Geometry: final body of the model. Coordinates: model frame, mm. A direction names the side the tool comes from. Give positions to 0.01 mm unless a question says otherwise; leave off trailing zeros. Write each loop counter-clockwise with the first axis right and the second up, starting at its lowest first coordinate (ties: lowest second). Pieces come first, ordered by that corner, then holes. Notation, with made-up numbers: (6.5, -7) -> (29.5, -7) arc R24 ccw to (29.5, 27) -> close; hole circle Ø2 at (11.5, -37.75). An arc over 180 degrees is marked (long way). Answer in a Markdown table with one row per item. Add a question column.
Item 1: Draft query along Y for faces 4 (the flat face through (-7.482, 2.799, 0.246)), 5 (the cylindrical face through (-7.956, 7.296, 0.682)), 6 (the flat face through (0, 0, 5)). Return one class per face: +Y half, -Y half, draft (parallel to the pull), parting line (faces both ways), or undercut.
Item 2: Material intervals for probe 1 along Z at (x, y) = (-5.25, 7.25); probe 2 along Z at (x, y) = (6, 2); probe 3 along X at (y, z) = (2.25, 3.9), sorted ascending. Write a range as from..to.
Item 3: Section query B-B on z = 3.6. Output: boundary loops of the cut face in (x, y).
Item 4: Section query A-A on y = 0. Output: boundary loops of the cut face in (x, z) (3 decimals), plus the area to 3 significant figures.
Item 5: First-contact query: P1, Ø1.5, axis at x = -5.5, y = -5, coming from the +Z side; P2, Ø11.5, axis at x = 4.5, y = -1, coming from the -Z side; P3, Ø1.5, axis at y = 2, z = 2, coming from the -X side; P4, Ø3, axis at x = -6.5, z = 0.5, coming from the +Y side. Flat tips, straight axial feed; report the tip coordinate or a pass-through.
Item 6: Access query for faces 1 (the flat face through (0, 0, 0)), 2 (the flat face through (-1.387, -4.757, 0.246)), 3 (the flat face through (2, -4, 2.5)). Directions: +Z, -Z, +X, -X, +Y, -Y. A direction counts if a zero-diameter tool reaches every point of the face in a straight line with its end or side. Return the directions, or none.
```python
from build123d import *

# Parameters (mm, degrees)
F0_R     = 4.064
F1_DEPTH = 5
F0_R_2   = 8.89
F2_DEPTH = 2.5
F0_R_3   = 10.795
F3_DEPTH = 1.5
F5_DEPTH = 0.5
F6_SIZE  = 0.508
F7_SIZE  = 0.381


with BuildPart() as f1:
    # F0 (on Top) → F1 (new body)
    with BuildSketch(Plane.XY):
        Circle(F0_R)
    extrude(amount=F1_DEPTH)

    # F0 (on Top) → F2 (join)
    with BuildSketch(Plane.XY):
        Circle(F0_R_2)
        Circle(F0_R, mode=Mode.SUBTRACT)
    extrude(amount=F2_DEPTH)

    # F0 (on Top) → F3 (join)
    with BuildSketch(Plane.XY):
        Circle(F0_R_3)
        Circle(F0_R_2, mode=Mode.SUBTRACT)
    extrude(amount=F3_DEPTH)

    # F4 (on face) → F5 (cut)
    with BuildSketch(Plane(origin=(0, 0, 0), x_dir=(1, 0, 0), z_dir=(0, 0, -1))):
        Polygon((-6.200742, -0.58), (-8.798818, -5.08), (-1.75, -5.08), (-1.75, -3.58), (-6.200742, -3.58), (-4.468691, -0.58), align=None)
        Polygon((0, 10.16), (-5.334716, 0.92), (-3.602666, 0.92), (-2.73664, 2.42), (0, 7.16), (1.870615, 3.92), (3.602666, 3.92), align=None)
        Polygon((1.75, -3.58), (1.75, -5.08), (8.798818, -5.08), (4.468691, 2.42), (2.73664, 2.42), (3.602666, 0.92), (6.200742, -3.58), align=None)
        Polygon((-2.73664, 2.42), (-3.602666, 0.92), (3.602666, 0.92), (2.73664, 2.42), align=None)
    extrude(amount=-F5_DEPTH, mode=Mode.SUBTRACT)

    # F6
    f6_edges = [f1.edges().sort_by_distance(p)[0] for p in [
        (-10.795, 0, 1.5),
    ]]
    chamfer(f6_edges, length=F6_SIZE)

    # F7
    f7_edges = [f1.edges().sort_by_distance(p)[0] for p in [
        (-10.795, 0, 0),
    ]]
    chamfer(f7_edges, length=F7_SIZE)


solid = f1.part
```
Findings below:
| question | item | result |
|---|---|---|
| 1 | face 4 | undercut |
| 1 | face 5 | parting line |
| 1 | face 6 | draft |
| 2 | probe 1 | z = 0..1.5 |
| 2 | probe 2 | z = 0.5..2.5 |
| 2 | probe 3 | x = -3.38..3.38 |
| 3 | outline | circle Ø8.13 at (0, 0) |
| 4 | outline | (-10.795, 0.381) -> (-10.414, 0) -> (4.134, 0) -> (4.134, 0.5) -> (5.866, 0.5) -> (5.866, 0) -> (10.414, 0) -> (10.795, 0.381) -> (10.795, 0.992) -> (10.287, 1.5) -> (8.89, 1.5) -> (8.89, 2.5) -> (4.064, 2.5) -> (4.064, 5) -> (-4.064, 5) -> (-4.064, 2.5) -> (-8.89, 2.5) -> (-8.89, 1.5) -> (-10.287, 1.5) -> (-10.795, 0.992) -> close |
| 4 | area | 69.2 mm^2 |
| 5 | P1 | stops at z = 2.5 |
| 5 | P2 | stops at z = 0 |
| 5 | P3 | stops at x = -10.36 |
| 5 | P4 | stops at y = 9.57 |
| 6 | face 1 | -Z, +X, -X, +Y, -Y |
| 6 | face 2 | -Z |
| 6 | face 3 | +Z |
